from build123d import *

# Parameters (mm, degrees)
ESQUISSE1_W                = 85
ESQUISSE1_H                = 50
BOSS_EXTRU_1_DEPTH         = 5
BOSS_EXTRU_2_START         = -14.3
BOSS_EXTRU_2_DEPTH         = 14.3
ESQUISSE3_R                = 3.5
ENL_V_MAT_EXTRU_1_DEPTH    = 14.3
R_P_TITION_LIN_AIRE2_COUNT = 2
R_P_TITION_LIN_AIRE2_PITCH = 24.9
BOSS_EXTRU_3_DEPTH         = 4.85
BOSS_EXTRU_3_DEPTH_BACK    = 4.85


# Read off the part's stored shape, not the designer's step: Boss.-Extru.2
with BuildPart() as part:
    # Esquisse1 → Boss.-Extru.1 (new body)
    with BuildSketch(Plane(origin=(0, 0, 0), x_dir=(1, 0, 0), z_dir=(0, 1, 0))):
        Rectangle(ESQUISSE1_W, ESQUISSE1_H)
    extrude(amount=BOSS_EXTRU_1_DEPTH)

    # Boss.-Extru.2 outline → Boss.-Extru.2 (add)
    with BuildSketch(Plane.ZY.offset(18.3).offset(BOSS_EXTRU_2_START)):
        with BuildLine():
            Line((25, 5), (25, 0.23226176))
            Line((25, 0.23226176), (25.260006787, -0.008238034))
            ThreePointArc((25.260006787, -0.008238034), (33.798445292, -3.53262012), (30.26, 5))
            Line((30.26, 5), (25, 5))
        make_face()
    boss_extru_2 = extrude(amount=BOSS_EXTRU_2_DEPTH)

    # Esquisse3 → Enlèv. mat.-Extru.1 (cut)
    with BuildSketch(Plane.ZY.offset(18.3)):
        with Locations((30.26, 0)):
            Circle(ESQUISSE3_R)
    enl_v_mat_extru_1 = extrude(amount=-ENL_V_MAT_EXTRU_1_DEPTH, mode=Mode.SUBTRACT)

    # Répétition linéaire2: Boss.-Extru.2, Enlèv. mat.-Extru.1 ×2
    with Locations(*[(i * R_P_TITION_LIN_AIRE2_PITCH, 0, 0) for i in range(1, R_P_TITION_LIN_AIRE2_COUNT)]):
        add(boss_extru_2)
        add(enl_v_mat_extru_1, mode=Mode.SUBTRACT)

    # Esquisse4 → Boss.-Extru.3 (add, two sides: drawn at the far end of the back side and taken through both)
    with BuildSketch(Plane(origin=(0, 0, 0), x_dir=(0, 0, -1), z_dir=(1, 0, 0)).offset(-BOSS_EXTRU_3_DEPTH_BACK)):
        with BuildLine():
            Line((26.5, 5), (25, 5))
            Line((25, 5), (25, -2.5))
            ThreePointArc((25, -2.5), (24.25, -3.25), (25, -4))
            Line((25, -4), (26.5, -4))
            Line((26.5, -4), (26.5, 5))
        make_face()
    extrude(amount=BOSS_EXTRU_3_DEPTH + BOSS_EXTRU_3_DEPTH_BACK)


solid = part.part
The model under review builds one solid part; all positions refer to its coordinate system, in mm. A direction names the side the tool comes from. Coordinates: 2 decimals unless noted, no trailing zeros. Loops run counter-clockwise (first coordinate to the right, second up) from the corner with the lowest first, then second, coordinate; pieces in that order, holes last. Notation, with made-up numbers: M 68,-27 L 73,-27 A14 ccw 73,-4 Z; hole C -16.75,38.5 d6. An arc over 180 degrees is marked long. Put each result on its own line as item: value. Start each with the question number.
Q1. Add section A-A (x = -7). Write out the cut boundary in (y, z), and give its area (3 significant figures).
Q2. Add section C-C (z = 5). Write out the cut boundary in (x, y).
Q3. Add section B-B (y = -1). Write out the cut boundary in (x, z), and give its area (3 significant figures).
Q4. Clearance check with flat-ended pins moving along their axes: pin 1 (1.1 mm diameter, centred on y = -0.5, z = -25, fed in from -X); pin 2 (1 mm diameter, centred on x = 29, y = 0.5, fed in from +Z); pin 3 (5 mm diameter, centred on y = 0.5, z = 31, fed in from +X); pin 4 (5.5 mm diameter, centred on x = -23, y = 3, fed in from -Z). State where each tip first meets the part, or that it passes through.
Q5. For faces 1 (the flat face through (6.6, 3.4, 28.9)), 2 (the flat face through (-18.3, 3.4, 28.9)), 3 (the flat face through (-1, 5, 1)), 4 (the flat face through (20.9, 3.4, 28.9)), 5 (the flat face through (-24, 2, -25)), list the 3-axis set-ups (+Z, -Z, +X, -X, +Y, -Y) from which the entire face can be reached by the end or side of a thin tool; tool diameter is ignored.
Q6. Wall thickness on line 1 (Y direction, x = -10, z = 30); line 2 (X direction, y = 2.25, z = 27); line 3 (Y direction, x = 28, z = 7): over which ranges is each line inside the solid? List them lowest first.
Q7. The part is to be moulded in two halves that separate along Z. For faces 6 (the flat face through (23, 2, -25)), 7 (the cylindrical face through (13.85, -3.65, 33.68)), 8 (the cylindrical face through (13.65, 0.154, 26.763)), 9 (the flat face through (-4, 3.4, 28.9)), say which applies: +Z half, -Z half, draft (parallel to the pull), parting line (faces both ways), or undercut.
Q8. Add section D-D (x = 36.5). Write out the cut boundary in (y, z).
Answers:
1. outline: M -0.01,25.26 L 0.23,25 L 0,25 L 0,-25 L 5,-25 L 5,30.26 A5 ccw long Z; hole C 0,30.26 d7
1. area: 297 mm^2
2. outline: M -42.5,0 L 42.5,0 L 42.5,5 L -42.5,5 Z
3. outline: M -18.3,25.36 L -4,25.36 L -4,26.91 L -18.3,26.91 Z; M -18.3,33.61 L -4,33.61 L -4,35.16 L -18.3,35.16 Z; M -4.85,-26.5 L 4.85,-26.5 L 4.85,-25 L -4.85,-25 Z; M 6.6,25.36 L 20.9,25.36 L 20.9,26.91 L 6.6,26.91 Z; M 6.6,33.61 L 20.9,33.61 L 20.9,35.16 L 6.6,35.16 Z
3. area: 103 mm^2
4. pin 1: stops at x = -42.5
4. pin 2: stops at z = 25
4. pin 3: passes through
4. pin 4: stops at z = -25
5. face 1: +Z, +Y, -Y
5. face 2: +Z, -X, +Y, -Y
5. face 3: +Z, -Z, +X, -X, +Y
5. face 4: +Z, +X, +Y, -Y
5. face 5: -Z, -X, +Y, -Y
6. line 1: y = -4.99 to -3.49, 3.49 to 5
6. line 2: x = -18.3 to -4, 6.6 to 20.9
6. line 3: y = 0 to 5
7. face 6: -Z half
7. face 7: parting line
7. face 8: undercut
7. face 9: draft
8. outline: M 0,-25 L 5,-25 L 5,25 L 0,25 Z
